```python
from build123d import *

# Parameters (mm, degrees)
F0_R     = 29.75
F1_DEPTH = 20
F2_R     = 8
F3_DEPTH = 15
F4_R     = 0.5
F5_R     = 3


with BuildPart() as f1:
    # F0 (on Top) → F1 (new body)
    with BuildSketch(Plane.XY):
        Circle(F0_R)
    extrude(amount=F1_DEPTH)

    # F2 (on face) → F3 (cut)
    with BuildSketch(Plane.XY.offset(20)):
        Circle(F2_R)
    extrude(amount=-F3_DEPTH, mode=Mode.SUBTRACT)

    # F4
    f4_edges = [f1.edges().sort_by_distance(p)[0] for p in [
        (-29.75, 0, 20),
    ]]
    fillet(f4_edges, radius=F4_R)

    # F5
    f5_edges = [f1.edges().sort_by_distance(p)[0] for p in [
        (-29.75, 0, 0),
    ]]
    fillet(f5_edges, radius=F5_R)


solid = f1.part
```
Here's how the part is built. I have some questions about the finished solid (model axes, mm). A direction names the side the tool comes from. Round coordinates to 2 decimals unless told otherwise and drop trailing zeros. Write each loop counter-clockwise with the first axis right and the second up, starting at its lowest first coordinate (ties: lowest second). Pieces come first, ordered by that corner, then holes.
Q1. If we section it at D-D on z = 3.75: Write out the boundary of the cut face in (x, y).
Q2. If we mould it in two halves opening along Y, with no side actions, what happens to faces 1 (the cylindrical face through (15.993, 25.085, 11.134)), 2 (the flat face through (0, 0, 0)), 3 (the flat face through (0, 0, 5))? For each: +Y half, -Y half, draft (parallel to the pull), parting line (faces both ways), or undercut.
Q3. Which directions (+Z, -Z, +X, -X, +Y, -Y) give clear straight access to the entire face, cutting with the end or side of a thin tool? Please do faces 4 (the cylindrical face through (-1.73, -7.81, 12.6)), 5 (the flat face through (6, -6, 20)).
Q4. Please list where these lines run through material, in increasing order: probe 1 along Y at (x, z) = (0, 8.25); probe 2 along X at (y, z) = (-7, 16.5); probe 3 along Y at (x, z) = (3, 17).
Q5. Will these pins go through, and if not, where does the flat tip stop? P1, Ø5, axis at x = 9, z = 12, coming from the +Y side; P2, Ø6, axis at x = -16.5, z = 9.5, coming from the +Y side; P3, Ø1.5, axis at x = -1.5, z = 6.5, coming from the +Y side; P4, Ø10, axis at y = 1, z = 11.5, coming from the +X side.
Q6. If we section it at C-C on z = 12.75: Write out the boundary of the cut face in (x, y).
Q7. If we section it at A-A on y = 0: Write out the boundary of the cut face in (x, z), plus the area to 3 significant figures.
Answer below:
1. outline: circle Ø59.5 at (0, 0)
2. face 1: parting line
2. face 2: draft
2. face 3: undercut
3. face 4: +Z
3. face 5: +Z, +X, -X, +Y, -Y
4. probe 1: y = -29.75 to -8, 8 to 29.75
4. probe 2: x = -28.91 to -3.87, 3.87 to 28.91
4. probe 3: y = -29.6 to -7.42, 7.42 to 29.6
5. P1: stops at y = 29.03
5. P2: stops at y = 26.51
5. P3: stops at y = 29.74
5. P4: stops at x = 29.75
6. outline: circle Ø59.5 at (0, 0); hole circle Ø16 at (0, 0)
7. outline: (-29.75, 3) arc R3 ccw to (-26.75, 0) - (26.75, 0) arc R3 ccw to (29.75, 3) - (29.75, 19.5) arc R0.5 ccw to (29.25, 20) - (8, 20) - (8, 5) - (-8, 5) - (-8, 20) - (-29.25, 20) arc R0.5 ccw to (-29.75, 19.5) - close
7. area: 946 mm2
